Source: CAD feature listing. Evaluate the final solid. Frame: model axes, mm. Face numbers are marked on the shaded views. A direction names the side the tool comes from. Give positions to 0.01 mm unless a question says otherwise; leave off trailing zeros. Loops run counter-clockwise (first coordinate to the right, second up) from the corner with the lowest first, then second, coordinate; pieces in that order, holes last. Notation, with made-up numbers: (-20, -33) -> (12, -33) arc R16 ccw to (12, -25) -> close; hole circle Ø1 at (-5.75, 54). An arc over 180 degrees is marked (long way). Answer as a JSON object with one key per item and string values. Group by question number.
Autodesk Inventor part; units mm, degrees
ref_plane "YZ Plane" through (0, 0, 0) normal (1, 0, 0) x (0, 1, 0)
ref_plane "XZ Plane" through (0, 0, 0) normal (0, 1, 0) x (-1, 0, 0)
ref_plane "XY Plane" through (0, 0, 0) normal (0, 0, 1) x (1, 0, 0)
sketch "スケッチ1" plane through (0, 0, 0) normal (0, 0, 1) x (1, 0, 0)
  line L0 (0, 0) -> (15, 0)
  line L1 (15, 0) -> (15, 15)
  line L2 (15, 15) -> (0, 15)
  line L3 (0, 15) -> (0, 0)
  dimension "d0" = 15
  dimension "d1" = 15
extrude "押し出し1" add sketch "スケッチ1" along normal blind 52.5
sketch "スケッチ2" plane through (0, 0, 52.5) normal (0, 0, 1) x (1, 0, 0)
  point P0 (0, 0)
sketch "スケッチ3" plane through (0, 0, 52.5) normal (0, 0, 1) x (1, 0, 0)
  line L0 (1, 1) -> (14, 1)
  line L1 (14, 1) -> (14, 14)
  line L2 (14, 14) -> (1, 14)
  line L3 (1, 14) -> (1, 1)
  line L4 (15, 15) -> (0, 15)
  line L5 (15, 0) -> (15, 15)
  point P0 (0, 0)
  dimension "d4" = 13
  dimension "d5" = 13
  dimension "d6" = 1
  dimension "d7" = 1
extrude "押し出し2" cut sketch "スケッチ3" against normal blind 52.5
sketch "スケッチ4" plane through (0, 15, 0) normal (0, 1, 0) x (1, 0, 0)
  circle A0 centre (7.5, -42.5) radius 1.6
  line L0 (15, -52.5) -> (0, -52.5)
  line L1 (15, 0) -> (15, -52.5)
  circle A1 centre (7.5, -10) radius 1.6
  line L2 (15, 0) -> (0, 0)
  circle A2 centre (7.5, -26.5) radius 1.6
  dimension "d10" = 3.2
  dimension "d11" = 10
  dimension "d12" = 7.5
  dimension "d13" = 3.2
  dimension "d14" = 10
  dimension "d15" = 7.5
  dimension "d16" = 3.2
  dimension "d17" = 16
  dimension "d18" = 16.5
hole "穴1" at (7.5, 15, 26.5) at (7.5, 15, 10) at (7.5, 15, 42.5) direction (0, -1, 0) diameter 3.2 depth 15
sketch "スケッチ5" plane through (0, 0, 52.5) normal (0, 0, 1) x (1, 0, 0)
  point P0 (0, 0)
  point P1 (7.773, 13.9735)
equation "\"BendRadius\" = Thickness"
equation "\"BendReliefWidth\" = Thickness"
equation "\"BendReliefDepth\" = 0.5 * Thickness"
equation "\"CornerReliefSize\" = 4 * Thickness"
equation "\"MinimumRemnant\" = 2 * Thickness"
equation "\"TransitionRadius\" = BendRadius"
equation "\"JacobiRadiusSize\" = BendRadius"
equation "\"GapSize\" = Thickness"
properties part number "足2"
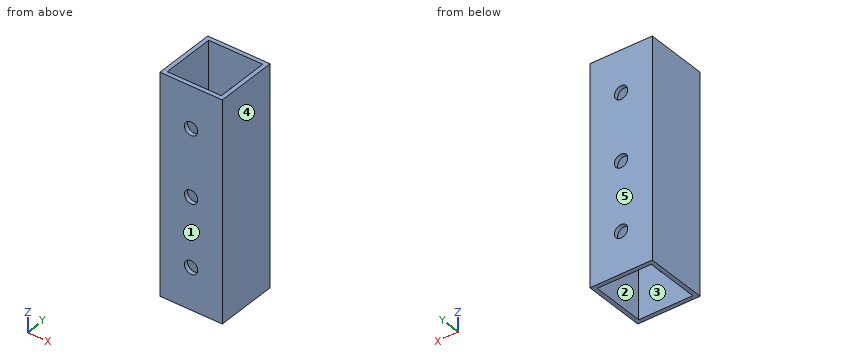
(1) Section query A-A on x = 7.5. State how many separate pieces and enclosed holes the cut face has, plus the area to 3 significant figures.
(2) Access query for the marked faces 1 and 2. Directions: +Z, -Z, +X, -X, +Y, -Y. A direction counts if a zero-diameter tool reaches every point of the face in a straight line with its end or side. Return the directions, or none.
(3) Section query B-B on z = 23.5. Return the cut outline in (x, y).
(4) Mould query, pull axis X, two halves, no side actions, for the marked faces 3, 4 and 5. Classes: pulls with the +X half, pulls with the -X half, needs draft (parallel to the pull), parting line crosses it, or undercut.
(5) Section query C-C on y = 10. Return the cut outline in (x, z), plus the area to 3 significant figures.
(6) Material intervals for line 1 (Z direction, x = 7.5, y = 0.6); line 2 (X direction, y = 8.5, z = 33), sorted ascending. Write a range as from..to.
(7) Section query D-D on z = 42.5. Return the cut outline in (x, y).
Result:
{
 "1": {"separate pieces": "8", "enclosed holes": "0", "area": "85.8 mm²"},
 "2": {"face 1": "+Z, -Z, +X, -X, -Y", "face 2": "+Z, -Z"},
 "3": {"outline": "(0, 0) -> (15, 0) -> (15, 15) -> (0, 15) -> close; hole (1, 1) -> (14, 1) -> (14, 14) -> (1, 14) -> close"},
 "4": {"face 3": "undercut", "face 4": "pulls with the +X half", "face 5": "needs draft"},
 "5": {"outline": "(0, 0) -> (1, 0) -> (1, 52.5) -> (0, 52.5) -> close; (14, 0) -> (15, 0) -> (15, 52.5) -> (14, 52.5) -> close", "area": "105 mm²"},
 "6": {"line 1": "0..8.4, 11.6..24.9, 28.1..40.9, 44.1..52.5", "line 2": "0..1, 14..15"},
 "7": {"outline": "(0, 0) -> (5.9, 0) -> (5.9, 1) -> (1, 1) -> (1, 14) -> (5.9, 14) -> (5.9, 15) -> (0, 15) -> close; (9.1, 0) -> (15, 0) -> (15, 15) -> (9.1, 15) -> (9.1, 14) -> (14, 14) -> (14, 1) -> (9.1, 1) -> close"}
}
